The listing builds one solid part. Answer for the finished solid, in the listing's coordinates (mm). Face numbers are marked on the shaded views. A direction names the side the tool comes from. Coordinates: 2 decimals unless noted, no trailing zeros. Write each loop counter-clockwise with the first axis right and the second up, starting at its lowest first coordinate (ties: lowest second). Pieces come first, ordered by that corner, then holes.
(1) For a pull along X with two mould halves and no side action, classify the marked faces 1, 2, 3 and 4 as +X half, -X half, draft (parallel to the pull), parting line (faces both ways), or undercut.
(2) Straight lines are drawn through the part: line 1 (X direction, y = 0.7, z = 0); line 2 (Y direction, x = -11.5, z = -7); line 3 (Y direction, x = 0.5, z = 12.75). For each, find the intervals that lie inside material, in ascending order.
(3) The part is cut by section C-C on y = 20. Determine the outline of the cut face in (x, z).
(4) Given P1, Ø3, axis at y = 18, z = -6.5, coming from the +X side; P2, Ø1.5, axis at x = -6.5, y = 19.5, coming from the +Z side; P3, Ø5.5, axis at x = -18.5, z = -5.5, coming from the -Y side, each flat-ended and moving along its own axis, determine where each tip first touches the part or whether it passes through.
(5) Which of the six approach directions +Z, -Z, +X, -X, +Y, -Y give full straight-line access (tool end or side, diameter ignored) to the marked faces 5, 6 and 7?
(6) The part is cut by section A-A on x = 0. Determine the outline of the cut face in (y, z), plus the area to 3 significant figures.
from build123d import *

# Parameters (mm, degrees)
SKETCH_1_R          = 15
EXTRUDE_1_DEPTH     = 17
SKETCH_2_R          = 11
EXTRUDE_2_DEPTH     = 1.5
SKETCH_3_R          = 15
EXTRUDE_3_DEPTH     = 3
SKETCH_4_R          = 11
EXTRUDE_4_DEPTH     = 4.5
SKETCH_6_W          = 44
SKETCH_6_H          = 30
EXTRUDE_6_DEPTH     = 33
SKETCH_7_W          = 5
SKETCH_7_H          = 30
EXTRUDE_7_DEPTH     = 2
SKETCH_9_R          = 13
SKETCH_9_R_2        = 12
CUT_EXTRUDE_2_DEPTH = 2


with BuildPart() as part:
    # 草圖1 → 伸長1 (new body)
    with BuildSketch(Plane(origin=(0, 0, 0), x_dir=(1, 0, 0), z_dir=(0, 1, 0))):
        with Locations(Location((0, 0, 0), (0, 0, 270))):
            Circle(SKETCH_1_R)
    extrude(amount=EXTRUDE_1_DEPTH)

    # 草圖2 → 伸長2 (add)
    with BuildSketch(Plane(origin=(0, 17, 0), x_dir=(1, 0, 0), z_dir=(0, 1, 0))):
        with Locations(Location((0, 0, 0), (0, 0, 270))):
            Circle(SKETCH_2_R)
    extrude(amount=EXTRUDE_2_DEPTH)

    # 草圖3 → 伸長3 (add)
    with BuildSketch(Plane(origin=(0, 18.5, 0), x_dir=(1, 0, 0), z_dir=(0, 1, 0))):
        with Locations(Location((0, 0, 0), (0, 0, 270))):
            Circle(SKETCH_3_R)
    extrude(amount=EXTRUDE_3_DEPTH)

    # 草圖4 → 伸長4 (add)
    with BuildSketch(Plane(origin=(0, 21.5, 0), x_dir=(1, 0, 0), z_dir=(0, 1, 0))):
        with Locations(Location((0, 0, 0), (0, 0, 270))):
            Circle(SKETCH_4_R)
    extrude(amount=EXTRUDE_4_DEPTH)

    # 草圖6 → 伸長6 (add)
    with BuildSketch(Plane(origin=(0, 26, 0), x_dir=(1, 0, 0), z_dir=(0, 1, 0))):
        Rectangle(SKETCH_6_W, SKETCH_6_H)
    extrude(amount=EXTRUDE_6_DEPTH)

    # 草圖7 → 伸長7 (add)
    with BuildSketch(Plane.XZ.offset(-26)):
        with Locations((-19.5, 0)):
            Rectangle(SKETCH_7_W, SKETCH_7_H)
    extrude(amount=EXTRUDE_7_DEPTH)

    # 草圖9 → 除料-伸長2 (cut)
    with BuildSketch(Plane.XZ):
        with Locations(Location((0, 0, 0), (0, 0, 270))):
            Circle(SKETCH_9_R)
        with Locations(Location((0, 0, 0), (0, 0, 270))):
            Circle(SKETCH_9_R_2, mode=Mode.SUBTRACT)
    extrude(amount=-CUT_EXTRUDE_2_DEPTH, mode=Mode.SUBTRACT)


solid = part.part
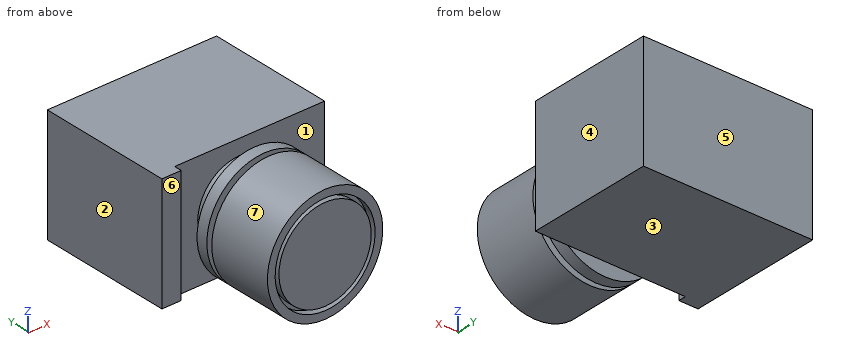
Model answer:
1. face 1: undercut
1. face 2: -X half
1. face 3: draft
1. face 4: +X half
2. line 1: x = -15 to -13, -12 to 12, 13 to 15
2. line 2: y = 0 to 17, 18.5 to 21.5, 26 to 59
2. line 3: y = 2 to 17, 18.5 to 21.5, 26 to 59
3. outline: circle Ø30 at (0, 0)
4. P1: stops at x = 14.11
4. P2: stops at z = 13.85
4. P3: stops at y = 24
5. face 5: +Z, -Z, +X, -X, +Y
5. face 6: +Z, -Z, -X, -Y
5. face 7: -Y
6. outline: (0, -15) - (17, -15) - (17, -11) - (18.5, -11) - (18.5, -15) - (21.5, -15) - (21.5, -11) - (26, -11) - (26, -15) - (59, -15) - (59, 15) - (26, 15) - (26, 11) - (21.5, 11) - (21.5, 15) - (18.5, 15) - (18.5, 11) - (17, 11) - (17, 15) - (0, 15) - (0, 13) - (2, 13) - (2, 12) - (0, 12) - (0, -12) - (2, -12) - (2, -13) - (0, -13) - close
6. area: 1,720 mm2
